```python
from build123d import *

# Parameters (mm, degrees)
SKETCH1_R           = 11
SKETCH1_R_2         = 9
BOSS_EXTRUDE1_DEPTH = 8
BOSS_EXTRUDE4_DEPTH = 8
CIRPATTERN2_COUNT   = 9


with BuildPart() as part:
    # Sketch1 → Boss-Extrude1 (new body)
    with BuildSketch(Plane(origin=(0, 0, 0), x_dir=(1, 0, 0), z_dir=(0, 1, 0))):
        with Locations(Location((0, 0, 0), (0, 0, 270))):
            Circle(SKETCH1_R)
        with Locations(Location((0, 0, 0), (0, 0, 270))):
            Circle(SKETCH1_R_2, mode=Mode.SUBTRACT)
    extrude(amount=BOSS_EXTRUDE1_DEPTH)

    # Sketch1<3> → Boss-Extrude4 (add)
    with BuildSketch(Plane(origin=(0, 0, 0), x_dir=(1, 0, 0), z_dir=(0, 1, 0))):
        with BuildLine():
            Line((-0.8, 18.469935747), (-0.8, 10.970870522))
            ThreePointArc((-0.8, 10.970870522), (0, 11), (0.8, 10.970870522))
            Line((0.8, 10.970870522), (0.8, 18.469935747))
            ThreePointArc((0.8, 18.469935747), (2.406716727, 18.329927471), (3.995116886, 18.050417379))
            Line((3.995116886, 18.050417379), (4.211218049, 19.026788357))
            ThreePointArc((4.211218049, 19.026788357), (0, 19.487253081), (-4.211218049, 19.026788357))
            Line((-4.211218049, 19.026788357), (-3.995116886, 18.050417379))
            ThreePointArc((-3.995116886, 18.050417379), (-2.406716727, 18.329927471), (-0.8, 18.469935747))
        make_face()
    boss_extrude4 = extrude(amount=BOSS_EXTRUDE4_DEPTH)

    # CirPattern2: Boss-Extrude4 ×9 about axis
    cirpattern2_axis = Axis((0, 0, 0), (0, 1, 0))
    for i in range(1, CIRPATTERN2_COUNT):
        add(boss_extrude4.rotate(cirpattern2_axis, i * 360 / CIRPATTERN2_COUNT))


solid = part.part
```
CAD build for the part. Positions are in the model's coordinates, mm. A direction names the side the tool comes from. Coordinates: 2 decimals unless noted, no trailing zeros. Write each loop counter-clockwise with the first axis right and the second up, starting at its lowest first coordinate (ties: lowest second). Pieces come first, ordered by that corner, then holes. Notation, with made-up numbers: (-37.5, 28.5) -> (-22.5, 28.5) arc R30 ccw to (-22.5, 57.5) -> close; hole circle Ø9 at (5.5, 0.25). An arc over 180 degrees is marked (long way). Return JSON: item names as keys, results as strings. Group by question number.
Q1. Flat gauge pins, fed straight in: pin 1 (12 mm diameter, centred on x = -7.5, z = 11, fed in from +Y); pin 2 (4 mm diameter, centred on x = 4.5, y = 3.5, fed in from -Z); pin 3 (2 mm diameter, centred on y = 3.5, z = -13.5, fed in from +X); pin 4 (4 mm diameter, centred on x = 5.5, z = -3, fed in from -Y). Where does each tip first touch, or does it go through?
Q2. Which spindle directions (+Z, -Z, +X, -X, +Y, -Y) get a long thin tool onto all of the face, cutting with end or side? Do faces 4 (the face through (17.086, 3.944, 7.06)), 5 (the face through (-6.7, 3.9, 18.3)), 6 (the face through (-10.19, 3.94, 16.01)). Say none if no direction does.
Q3. Pull direction Z, two halves, no side cores. Call faces 1 (the face through (14.58, 3.94, -1.76)), 2 (the face through (16.847, 3.944, 9.795)), 3 (the face through (-8.77, 3.94, -16.83)): released by +Z, released by -Z, zero draft, split by the parting line, or undercut.
Q4. Cut at A-A, the plane x = 0. Give the cut face in (y, z).
Q5. Drill centre lines: line 1 (X direction, y = 1.5, z = 0); line 2 (X direction, y = 6.25, z = -11); line 3 (X direction, y = 0.75, z = 12). Where is each one in solid material? Low to high.
Q6. Cut at C-C, the plane z = 15. Give the cut face in (x, y), then the cut area to 3 significant figures.
Q7. Cut at B-B, the plane z = 0. Give the cut face in (x, y).
Returned:
{
 "1": {"pin 1": "stops at y = 8", "pin 2": "stops at z = -19.33", "pin 3": "stops at x = 14.95", "pin 4": "passes through"},
 "2": {"face 4": "+Y, -Y", "face 5": "+Z, -X, +Y, -Y", "face 6": "-X, +Y, -Y"},
 "3": {"face 1": "undercut", "face 2": "released by +Z", "face 3": "released by -Z"},
 "4": {"outline": "(0, -19.49) -> (8, -19.49) -> (8, -9) -> (0, -9) -> close; (0, 9) -> (8, 9) -> (8, 11) -> (0, 11) -> close"},
 "5": {"line 1": "x = -19.49 to -18.49, -11 to -9, 9 to 11, 18.49 to 19.49", "line 2": "x = -10.27 to -8.19, -0.8 to 0.8, 8.19 to 10.27", "line 3": "x = -15.35 to -14.06, -5.22 to -3.52, 3.52 to 5.22, 14.06 to 15.35"},
 "6": {"outline": "(-6.31, 0) -> (-4.61, 0) -> (-4.61, 8) -> (-6.31, 8) -> close; (4.61, 0) -> (6.31, 0) -> (6.31, 8) -> (4.61, 8) -> close", "area": "27.2 mm2"},
 "7": {"outline": "(-19.49, 0) -> (-18.49, 0) -> (-18.49, 8) -> (-19.49, 8) -> close; (-11, 0) -> (-9, 0) -> (-9, 8) -> (-11, 8) -> close; (9, 0) -> (11, 0) -> (11, 8) -> (9, 8) -> close; (18.49, 0) -> (19.49, 0) -> (19.49, 8) -> (18.49, 8) -> close"}
}
